For this review, use the dimensioned drawing (mm, ordinates from the lowest corner) and the shaded views. Give positions to 0.01 mm unless a question says otherwise; leave off trailing zeros. Write each loop counter-clockwise with the first axis right and the second up, starting at its lowest first coordinate (ties: lowest second). Pieces come first, ordered by that corner, then holes.
1) Wall thickness on line 1 along X through (y, z) = (5, 11.75) (1 decimal); line 2 along Y through (x, z) = (5.5, 8) (1 decimal); line 3 along X through (y, z) = (3, 8.75) (1 decimal): over which ranges is each line inside the solid? List them lowest first.
2) For P1, Ø2, axis at x = 8, y = 8, coming from the -Z side; P2, Ø4, axis at y = 2, z = 2.5, coming from the +X side; P3, Ø1, axis at x = 2.5, z = 5, coming from the -Y side; P4, Ø1.5, axis at x = 8, z = 7, coming from the +Y side (1 decimal), all flat-tipped, find the tip position at first contact; note any pin that passes through.
3) We need section A-A on z = 5.25. Give the boundary of the cut face in (x, y) (1 decimal).
4) Draft analysis for pull direction X (two halves, no side actions). For the marked faces 1, 2 and 3, state which applies: pulls with the +X half, pulls with the -X half, needs draft (parallel to the pull), parting line crosses it, or undercut.
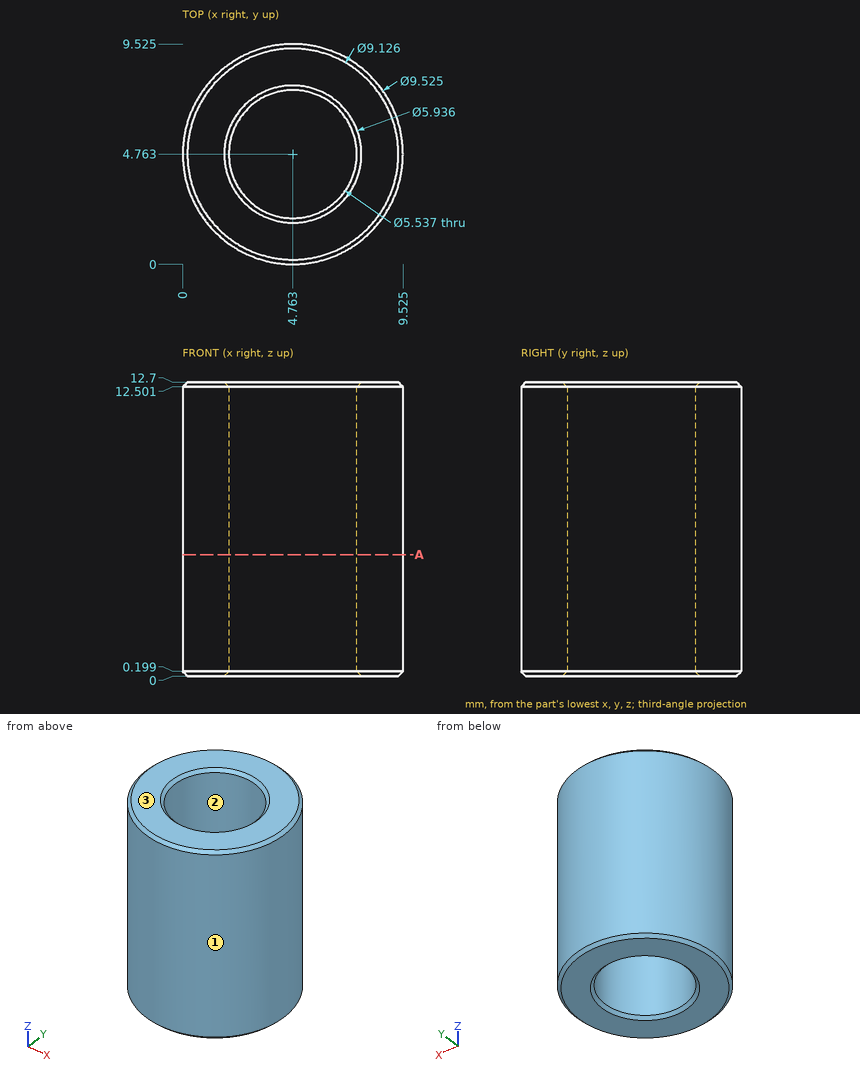
Results list:
1. line 1: x = 0 to 2, 7.5 to 9.5
1. line 2: y = 0.1 to 2.1, 7.4 to 9.5
1. line 3: x = 0.3 to 2.6, 6.9 to 9.2
2. P1: stops at z = 0
2. P2: stops at x = 9.46
2. P3: stops at y = 0.34
2. P4: stops at y = 8.8
3. outline: circle Ø9.5 at (4.8, 4.8); hole circle Ø5.5 at (4.8, 4.8)
4. face 1: parting line crosses it
4. face 2: undercut
4. face 3: needs draft
